Can you work these out from the model? Positions are in its coordinate system, mm. Round coordinates to 2 decimals unless told otherwise and drop trailing zeros. Order: outer loops, then holes, each group sorted by start corner. A loop starts at its lowest first (then second) coordinate and runs counter-clockwise, first axis right, second up.
Q1. If we section it at B-B (x = 0): Please give me the cut outline in (y, z).
Q2. If I drill on line 1 (Z direction, x = 0, y = 1.4); line 2 (Z direction, x = -1.75, y = 0.35); line 3 (X direction, y = 0.85, z = -2), over which ranges is the centre line in solid material (lowest first)?
Q3. If we section it at A-A (z = 0): Please give me the cut outline in (x, y).
Q4. If we section it at C-C (y = 0.7): Please give me the cut outline in (x, z).
Q5. We'd pull the mould along Z, two halves only. Please class faces 1 (the face through (-5.96, 1.14, 1.88)), 2 (the face through (-2.285, 1.482, 3.584)), 3 (the face through (-1.4, 0, 4.5)): pulls with the +Z half, pulls with the -Z half, needs draft (parallel to the pull), parting line crosses it, or undercut.
from build123d import *

# Parameters (mm, degrees)
CHAMFER1_SIZE = 0.25


with BuildPart() as part:
    # Sketch1 → Revolve1 (revolve)
    with BuildSketch(Plane.XY):
        Polygon((-4.25, 3), (-4.25, 0), (-6.25, 0), (-6.25, 2), (-4.75, 3), align=None)
    revolve(axis=Axis((0, 0, 0), (0, 1, 0)))

    # Chamfer1
    chamfer1_edges = [part.edges().sort_by_distance(p)[0] for p in [
        (6.25, 0, 0),
        (4.25, 0, 0),
        (4.25, 3, 0),
    ]]
    chamfer(chamfer1_edges, length=CHAMFER1_SIZE)


solid = part.part
Solution:
1. outline: (0, -6) - (0.25, -6.25) - (2, -6.25) - (3, -4.75) - (3, -4.5) - (2.75, -4.25) - (0.25, -4.25) - (0, -4.5) - close; (0, 4.5) - (0.25, 4.25) - (2.75, 4.25) - (3, 4.5) - (3, 4.75) - (2, 6.25) - (0.25, 6.25) - (0, 6) - close
2. line 1: z = -6.25 to -4.25, 4.25 to 6.25
2. line 2: z = -6 to -3.87, 3.87 to 6
2. line 3: x = -5.92 to -3.75, 3.75 to 5.92
3. outline: (-6.25, 0.25) - (-6, 0) - (-4.5, 0) - (-4.25, 0.25) - (-4.25, 2.75) - (-4.5, 3) - (-4.75, 3) - (-6.25, 2) - close; (4.25, 0.25) - (4.5, 0) - (6, 0) - (6.25, 0.25) - (6.25, 2) - (4.75, 3) - (4.5, 3) - (4.25, 2.75) - close
4. outline: circle Ø12.5 at (0, 0); hole circle Ø8.5 at (0, 0)
5. face 1: parting line crosses it
5. face 2: undercut
5. face 3: needs draft
